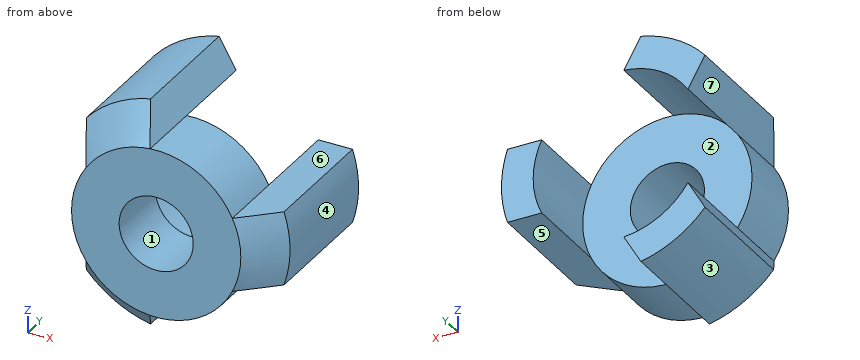
```python
from build123d import *

# Parameters (mm, degrees)
F0_R        = 101.6
F0_R_2      = 44.45
F1_DEPTH    = 79.375
F3_DEPTH    = 187.452
F4_SIZE     = 38.1
F5_T2_ANGLE = 117.4823583848
F6_T2_ANGLE = 117.4823583848


# Not quite as in the source:
# - a fillet or chamfer that OpenCascade refuses, or shapes differently, is made with other operations: its cross-section is extruded or revolved along the edge and cut away or added


with BuildPart() as f1:
    # F0 (on Front) → F1 (new body)
    with BuildSketch(Plane.XZ):
        Circle(F0_R)
        Circle(F0_R_2, mode=Mode.SUBTRACT)
    extrude(amount=F1_DEPTH)

    # F2 (on face) → F3 (join)
    with BuildSketch(Plane.XZ.offset(79.375)):
        with BuildLine():
            Line((132.4397504528, 44.45), (91.3605905191, 44.45))
            ThreePointArc((91.3605905191, 44.45), (101.6, 0), (91.3605905191, -44.45))
            Line((91.3605905191, -44.45), (132.4397504528, -44.45))
            ThreePointArc((132.4397504528, -44.45), (139.7, 0), (132.4397504528, 44.45))
        make_face()
        with BuildLine():
            Line((-104.7147044246, 92.471188363), (-84.1751244578, 56.8955922943))
            ThreePointArc((-84.1751244578, 56.8955922943), (-50.8, 87.9881810245), (-7.1854660613, 101.3455922943))
            Line((-7.1854660613, 101.3455922943), (-27.7250460282, 136.921188363))
            ThreePointArc((-27.7250460282, 136.921188363), (-69.85, 120.9837489087), (-104.7147044246, 92.471188363))
        make_face()
        with BuildLine():
            Line((-27.7250460282, -136.921188363), (-7.1854660613, -101.3455922943))
            ThreePointArc((-7.1854660613, -101.3455922943), (-50.8, -87.9881810245), (-84.1751244578, -56.8955922943))
            Line((-84.1751244578, -56.8955922943), (-104.7147044246, -92.471188363))
            ThreePointArc((-104.7147044246, -92.471188363), (-69.85, -120.9837489087), (-27.7250460282, -136.921188363))
        make_face()
    extrude(amount=-F3_DEPTH)

    # F4
    f4_edges = [f1.edges().sort_by_distance(p)[0] for p in [
        (139.7, -79.375, 0),
    ]]
    chamfer(f4_edges, length=F4_SIZE)

    # F5: chamfer of 38.1 on 1 edges, made by hand

    # F5_s1 → F5_t2 (revolve, cut)
    with BuildSketch(Plane(origin=(0, 0, 0), x_dir=(0, 1, 0), z_dir=(-0.0219688003, 0, 0.9997586568))):
        Polygon((-79.375, 101.6), (-41.275, 139.7), (-79.375, 139.7), align=None)
    revolve(axis=Axis((0, -79.375, 0), (0, -1, 0)), revolution_arc=F5_T2_ANGLE, mode=Mode.SUBTRACT)

    # F6: chamfer of 38.1 on 1 edges, made by hand

    # F6_s1 → F6_t2 (revolve, cut)
    with BuildSketch(Plane(origin=(0, 0, 0), x_dir=(0, 1, 0), z_dir=(0.8768007946, 0, -0.4808537893))):
        Polygon((-79.375, 101.6), (-41.275, 139.7), (-79.375, 139.7), align=None)
    revolve(axis=Axis((0, -79.375, 0), (0, -1, 0)), revolution_arc=F6_T2_ANGLE, mode=Mode.SUBTRACT)


solid = f1.part
```
Check sheet for the modelled part. Datum: model origin and axes. Units: mm. Face numbers are marked on the shaded views. A direction names the side the tool comes from. Coordinates: 2 decimals unless noted, no trailing zeros. Write each loop counter-clockwise with the first axis right and the second up, starting at its lowest first coordinate (ties: lowest second). Pieces come first, ordered by that corner, then holes. Notation, with made-up numbers: (10.5, 77) -> (40.5, 77) arc R9 cw to (40.5, 87) -> close; hole circle Ø5 at (54, -11). An arc over 180 degrees is marked (long way). Use a Markdown table: item, result.
1. Release check for a two-part mould opening along X. For the marked faces 1, 2, 3 and 4 record: pulls with the +X half, pulls with the -X half, needs draft (parallel to the pull), parting line crosses it, or undercut.
Reported:
| item | result |
|---|---|
| face 1 | undercut |
| face 2 | needs draft |
| face 3 | pulls with the -X half |
| face 4 | pulls with the +X half |
2. Tool access check on the marked faces 5, 6 and 7. Record the directions out of +Z, -Z, +X, -X, +Y, -Y that give a thin tool (end or side, any length) a straight path to the whole face; none if there is none.
Reported:
| item | result |
|---|---|
| face 5 | -Z, +X, +Y, -Y |
| face 6 | +Z, +X, +Y, -Y |
| face 7 | -X, +Y, -Y |
3. Scan lines: line 1 along Z through (x, y) = (0, -20); line 2 along X through (y, z) = (-8.5, 2); line 3 along Y through (x, z) = (49.5, 71) (3 decimals). Record each from-to range of solid material in increasing order.
Reported:
| item | result |
|---|---|
| line 1 | z = -101.6 to -44.45, 44.45 to 101.6 |
| line 2 | x = -101.58 to -44.4, 44.4 to 139.69 |
| line 3 | y = -79.375 to 0 |
4. Sectioned sample at D-D (y = 77.5). Enter the section's corners in (x, z), plus the area to 3 significant figures.
Reported:
| item | result |
|---|---|
| outline | (-104.71, -92.47) arc R139.7 ccw to (-27.73, -136.92) -> (-7.19, -101.35) arc R101.6 cw to (-84.18, -56.9) -> close; (-104.71, 92.47) -> (-84.18, 56.9) arc R101.6 cw to (-7.19, 101.35) -> (-27.73, 136.92) arc R139.7 ccw to start; (91.36, -44.45) -> (132.44, -44.45) arc R139.7 ccw to (132.44, 44.45) -> (91.36, 44.45) arc R101.6 cw to start |
| area | 10,400 mm2 |
5. Sectioned sample at B-B (z = 0). Enter the section's corners in (x, y) (3 decimals), plus the area to 3 significant figures.
Reported:
| item | result |
|---|---|
| outline | (-101.6, -79.375) -> (-44.45, -79.375) -> (-44.45, 0) -> (-101.6, 0) -> close; (44.45, -79.375) -> (101.6, -79.375) -> (139.7, -41.275) -> (139.7, 108.077) -> (101.6, 108.077) -> (101.6, 0) -> (44.45, 0) -> close |
| area | 15,500 mm2 |
6. Sectioned sample at C-C (x = 0). Enter the section's corners in (y, z) (3 decimals).
Reported:
| item | result |
|---|---|
| outline | (-79.375, -101.6) -> (0, -101.6) -> (0, -44.45) -> (-79.375, -44.45) -> close; (-79.375, 44.45) -> (0, 44.45) -> (0, 101.6) -> (-79.375, 101.6) -> close |
7. Go/stop test with flat-tipped pins: pin 1 Ø12 at (y, z) = (54.5, 35) entering from +X; pin 2 Ø4 at (y, z) = (-9, 43) entering from +X; pin 3 Ø12.5 at (x, y) = (118, 0.5) entering from +Z. Record where each tip stops, or that it passes through.
Reported:
| item | result |
|---|---|
| pin 1 | stops at x = 136.66 |
| pin 2 | stops at x = 133.55 |
| pin 3 | stops at z = 44.45 |
8. Sectioned sample at A-A (y = -37). Enter the section's corners in (x, z), plus the area to 3 significant figures.
Reported:
| item | result |
|---|---|
| outline | (-104.71, -92.47) arc R139.7 ccw to (-27.73, -136.92) -> (-7.19, -101.35) arc R101.6 ccw to (91.36, -44.45) -> (132.44, -44.45) arc R139.7 ccw to (132.44, 44.45) -> (91.36, 44.45) arc R101.6 ccw to (-7.19, 101.35) -> (-27.73, 136.92) arc R139.7 ccw to (-104.71, 92.47) -> (-84.18, 56.9) arc R101.6 ccw to (-84.18, -56.9) -> close; hole circle Ø88.9 at (0, 0) |
| area | 36,600 mm2 |
